```python
from build123d import *

# Parameters (mm, degrees)
SKETCH1_W           = 120
SKETCH1_H           = 80
BOSS_EXTRUDE1_DEPTH = 10
SKETCH2_W           = 20
SKETCH2_H           = 40
CUT_EXTRUDE1_DEPTH  = 11
FILLET1_R           = 10
FILLET2_R           = 5


with BuildPart() as part:
    # Sketch1 → Boss-Extrude1 (new body)
    with BuildSketch(Plane.XZ.offset(150)):
        with Locations((-26.489460092, -13.07873573)):
            Rectangle(SKETCH1_W, SKETCH1_H)
    extrude(amount=BOSS_EXTRUDE1_DEPTH)

    # Sketch2 → Cut-Extrude1 (cut, through all)
    with BuildSketch(Plane(origin=(0, -150, 0), x_dir=(1, 0, 0), z_dir=(0, 1, 0))):
        with Locations((-76.489460092, 13.07873573)):
            Rectangle(SKETCH2_W, SKETCH2_H)
    extrude(amount=-CUT_EXTRUDE1_DEPTH, mode=Mode.SUBTRACT)

    # Fillet1
    fillet1_edges = [part.edges().sort_by_distance(p)[0] for p in [
        (-66.489460092, -155, -33.07873573),
        (-66.489460092, -155, 6.92126427),
    ]]
    fillet(fillet1_edges, radius=FILLET1_R)

    # Fillet2
    fillet2_edges = [part.edges().sort_by_distance(p)[0] for p in [
        (-86.489460092, -155, 6.92126427),
        (-86.489460092, -155, -33.07873573),
    ]]
    fillet(fillet2_edges, radius=FILLET2_R)


solid = part.part
```
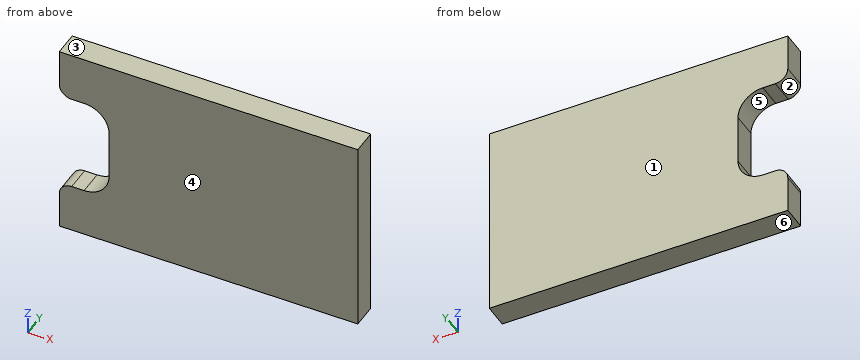
Verification items for the finished model (mm, model axes). Face numbers are marked on the shaded views. A direction names the side the tool comes from. Coordinates: 2 decimals unless noted, no trailing zeros. Loops run counter-clockwise (first coordinate to the right, second up) from the corner with the lowest first, then second, coordinate; pieces in that order, holes last. Notation, with made-up numbers: (56.25, 73) -> (95.25, 73) arc R14 cw to (95.25, 95) -> close; hole circle Ø9 at (-11, 63.25). An arc over 180 degrees is marked (long way). Answer in a Markdown table with one row per item. Add a question column.
1. Section check A-A, the plane y = -153.5. Enter the section's corners in (x, z).
2. Section check C-C, the plane z = -26. Enter the section's corners in (x, y), then the cut area to 3 significant figures.
3. Section check B-B, the plane z = -11.5. Enter the section's corners in (x, y), then the cut area to 3 significant figures.
4. Material ranges on probe 1 along X at (y, z) = (-153.25, -8.5); probe 2 along Z at (x, y) = (-72.5, -153); probe 3 along X at (y, z) = (-151, 10.5), recorded low to high. Write a range as [from, to].
5. Access from +Z, -Z, +X, -X, +Y, -Y to the whole of each face (thin tool, end or side, straight path). Record for the marked faces 1 and 2.
6. Draft check along Z on the marked faces 3, 4, 5 and 6. Enter one of: +Z half, -Z half, draft (parallel to the pull), parting line (faces both ways), or undercut.
Derived:
| question | item | result |
|---|---|---|
| 1 | outline | (-86.49, -53.08) -> (33.51, -53.08) -> (33.51, 26.92) -> (-86.49, 26.92) -> (-86.49, 11.92) arc R5 ccw to (-81.49, 6.92) -> (-76.49, 6.92) arc R10 cw to (-66.49, -3.08) -> (-66.49, -23.08) arc R10 cw to (-76.49, -33.08) -> (-81.49, -33.08) arc R5 ccw to (-86.49, -38.08) -> close |
| 2 | outline | (-66.93, -160) -> (33.51, -160) -> (33.51, -150) -> (-66.93, -150) -> close |
| 2 | area | 1,000 mm² |
| 3 | outline | (-66.49, -160) -> (33.51, -160) -> (33.51, -150) -> (-66.49, -150) -> close |
| 3 | area | 1,000 mm² |
| 4 | probe 1 | x = [-66.49, 33.51] |
| 4 | probe 2 | z = [-53.08, -32.25], [6.09, 26.92] |
| 4 | probe 3 | x = [-86.28, 33.51] |
| 5 | face 1 | +Z, -Z, +X, -X, +Y |
| 5 | face 2 | -X, +Y, -Y |
| 6 | face 3 | +Z half |
| 6 | face 4 | draft |
| 6 | face 5 | undercut |
| 6 | face 6 | -Z half |
